Geometry check sheet. Reference: the model listing, model coordinates, mm. Face numbers are marked on the shaded views. A direction names the side the tool comes from. Give positions to 0.01 mm unless a question says otherwise; leave off trailing zeros. Loops run counter-clockwise (first coordinate to the right, second up) from the corner with the lowest first, then second, coordinate; pieces in that order, holes last.
```python
from build123d import *

# Parameters (mm, degrees)
SKETCH1_R                      = 9.525
BOSS_EXTRUDE1_DEPTH            = 80.9625
SKETCH2_R                      = 19.05
BOSS_EXTRUDE2_DEPTH            = 4.7498
SKETCH5_OUTSIDE_W              = 60.348
SKETCH5_OUTSIDE_H              = 60.348
SKETCH5_OUTSIDE_R              = 8.4328
CUT_EXTRUDE1_DEPTH             = 12.954
SKETCH7_R                      = 12.7
BOSS_EXTRUDE3_DEPTH            = 3.175
F_8_32_TAPPED_HOLE1_AT_2_COUNT = 2
F_8_32_TAPPED_HOLE1_AT_2_PITCH = 12.7
F_8_32_TAPPED_HOLE1_AT_3_COUNT = 2
F_8_32_TAPPED_HOLE1_AT_3_PITCH = 21.997045256
F_8_32_TAPPED_HOLE1_AT_4_COUNT = 2
F_8_32_TAPPED_HOLE1_AT_4_PITCH = 25.4
F_8_32_TAPPED_HOLE1_AT_5_COUNT = 2
F_8_32_TAPPED_HOLE1_AT_5_PITCH = 21.997045256
F_8_32_TAPPED_HOLE1_AT_6_COUNT = 2
F_8_32_TAPPED_HOLE1_AT_6_PITCH = 12.7
SKETCH6_R                      = 6.35
CUT_EXTRUDE2_DEPTH             = 90.846554588
SKETCH10_R                     = 9.525
SKETCH10_R_2                   = 6.35
BOSS_EXTRUDE4_DEPTH            = 47.625
F_5_8_11_TAPPED_HOLE1_D        = 13.49248
F_5_8_11_TAPPED_HOLE1_DEPTH    = 25.4
F_5_8_11_TAPPED_HOLE1_TIP      = 4.053549943
CUT_EXTRUDE3_DEPTH             = 1.5875
FILLET1_R                      = 0.79375
CHAMFER1_SIZE                  = 0.254


with BuildPart() as part:
    # Sketch1 → Boss-Extrude1 (new body)
    with BuildSketch(Plane.XY):
        Circle(SKETCH1_R)
    extrude(amount=BOSS_EXTRUDE1_DEPTH)

    # Sketch2 → Boss-Extrude2 (add)
    with BuildSketch(Plane.XY.offset(80.9625)):
        Circle(SKETCH2_R)
    extrude(amount=BOSS_EXTRUDE2_DEPTH)

    # Sketch5 outside → Cut-Extrude1 (cut)
    with BuildSketch(Plane(origin=(0, 0, 0), x_dir=(-1, 0, 0), z_dir=(0, 0, -1))):
        Rectangle(SKETCH5_OUTSIDE_W, SKETCH5_OUTSIDE_H)
        Circle(SKETCH5_OUTSIDE_R, mode=Mode.SUBTRACT)
    extrude(amount=-CUT_EXTRUDE1_DEPTH, mode=Mode.SUBTRACT)

    # Sketch7 → Boss-Extrude3 (add)
    with BuildSketch(Plane(origin=(0, 0, 71.4375), x_dir=(-1, 0, 0), z_dir=(0, 0, -1))):
        Circle(SKETCH7_R)
    extrude(amount=BOSS_EXTRUDE3_DEPTH)

    # Sketch8 → #8-32 Tapped Hole1 (revolve, cut)
    with BuildSketch(Plane(origin=(0, 12.7, 80.9625), x_dir=(0, 1, 0), z_dir=(1, 0, 0))):
        Polygon((0, 0), (0, 11.705806461), (1.7272, 10.668), (1.7272, 0), align=None)
    f_8_32_tapped_hole1 = revolve(axis=Axis((0, 12.7, 74.6125), (0, 0, 1)), mode=Mode.SUBTRACT)

    # #8-32 Tapped Hole1 at 2: #8-32 Tapped Hole1 ×2
    with Locations(*[Vector(-0.8660254037844382, -0.500000000000001, 0) * (i * F_8_32_TAPPED_HOLE1_AT_2_PITCH) for i in range(1, F_8_32_TAPPED_HOLE1_AT_2_COUNT)]):
        add(f_8_32_tapped_hole1, mode=Mode.SUBTRACT)

    # #8-32 Tapped Hole1 at 3: #8-32 Tapped Hole1 ×2
    with Locations(*[Vector(-0.5000000000000153, -0.8660254037844298, 0) * (i * F_8_32_TAPPED_HOLE1_AT_3_PITCH) for i in range(1, F_8_32_TAPPED_HOLE1_AT_3_COUNT)]):
        add(f_8_32_tapped_hole1, mode=Mode.SUBTRACT)

    # #8-32 Tapped Hole1 at 4: #8-32 Tapped Hole1 ×2
    with Locations(*[(0, -i * F_8_32_TAPPED_HOLE1_AT_4_PITCH, 0) for i in range(1, F_8_32_TAPPED_HOLE1_AT_4_COUNT)]):
        add(f_8_32_tapped_hole1, mode=Mode.SUBTRACT)

    # #8-32 Tapped Hole1 at 5: #8-32 Tapped Hole1 ×2
    with Locations(*[Vector(0.4999999999999846, -0.8660254037844476, 0) * (i * F_8_32_TAPPED_HOLE1_AT_5_PITCH) for i in range(1, F_8_32_TAPPED_HOLE1_AT_5_COUNT)]):
        add(f_8_32_tapped_hole1, mode=Mode.SUBTRACT)

    # #8-32 Tapped Hole1 at 6: #8-32 Tapped Hole1 ×2
    with Locations(*[Vector(0.86602540378443, -0.5000000000000151, 0) * (i * F_8_32_TAPPED_HOLE1_AT_6_PITCH) for i in range(1, F_8_32_TAPPED_HOLE1_AT_6_COUNT)]):
        add(f_8_32_tapped_hole1, mode=Mode.SUBTRACT)

    # Sketch6 → Cut-Extrude2 (cut, through all)
    with BuildSketch(Plane(origin=(0, 0, 0), x_dir=(-1, 0, 0), z_dir=(0, 0, -1))):
        Circle(SKETCH6_R)
    extrude(amount=-CUT_EXTRUDE2_DEPTH, mode=Mode.SUBTRACT)

    # Sketch10 → Boss-Extrude4 (add)
    with BuildSketch(Plane.XY.offset(85.7123)):
        with Locations(Location((0, 0, 0), (0, 0, 180))):
            Circle(SKETCH10_R)
        with Locations(Location((0, 0, 0), (0, 0, 180))):
            Circle(SKETCH10_R_2, mode=Mode.SUBTRACT)
    extrude(amount=BOSS_EXTRUDE4_DEPTH)

    # 5/8-11 Tapped Hole1
    with Locations(Plane.XY.offset(133.3373)):
        with Locations((0, 0)):
            Hole(F_5_8_11_TAPPED_HOLE1_D / 2, depth=F_5_8_11_TAPPED_HOLE1_DEPTH)
            with Locations((0, 0, -(F_5_8_11_TAPPED_HOLE1_DEPTH + F_5_8_11_TAPPED_HOLE1_TIP / 2))):  # 118° drill point
                Cone(0, F_5_8_11_TAPPED_HOLE1_D / 2, F_5_8_11_TAPPED_HOLE1_TIP, mode=Mode.SUBTRACT)

    # Sketch13 → Cut-Extrude3 (cut)
    with BuildSketch(Plane(origin=(0, 0, 0), x_dir=(-1, 0, 0), z_dir=(0, 0, -1))):
        with BuildLine():
            Line((-0.79375, -6.604), (-0.79375, 6.604))
            ThreePointArc((-0.79375, 6.604), (0, 7.39775), (0.79375, 6.604))
            Line((0.79375, 6.604), (0.79375, -6.604))
            ThreePointArc((0.79375, -6.604), (0, -7.39775), (-0.79375, -6.604))
        make_face()
    extrude(amount=-CUT_EXTRUDE3_DEPTH, mode=Mode.SUBTRACT)

    # Fillet1
    # the kernel refuses this fillet: 0.79375 mm, written as the material it takes off along each edge
    with BuildSketch(Plane(origin=(0.79375, -6.300195309, 1.5875), x_dir=(0.9853201649720871, 0.17071664388506244, 0), z_dir=(0, 0, -1)), Plane(origin=(-0.79375, 6.300195309, 1.5875), x_dir=(-0.9853201649720869, -0.17071664388506383, 0), z_dir=(0, 0, -1))) as fillet1_piece_1:
        with BuildLine():
            CenterArc((0.623581926, 0.792901977), FILLET1_R, 203.344606785, 64.006660147)
            Line((-0.105190236, 0.478370264), (-0.178067452, 0.446917093))
            ThreePointArc((-0.178067452, 0.446917093), (-0.130074305, 0.285794254), (-0.078209788, -0.013550634))
            Line((-0.078209788, -0.013550634), (0.003668129, -0.079290198))
            ThreePointArc((0.003668129, -0.079290198), (0.293450318, -0.072590818), (0.583232507, -0.079290198))
            Line((0.583232507, -0.079290198), (0.586900636, 0))
        make_face()
    extrude(amount=3.054751591, mode=Mode.SUBTRACT)
    with BuildSketch(Plane(origin=(0.79375, 6.300195309, 1.5875), x_dir=(0.985320164972087, -0.17071664388506264, 0), z_dir=(0, 0, -1)), Plane(origin=(-0.79375, -6.300195309, 1.5875), x_dir=(-0.9853201649720869, 0.17071664388506363, 0), z_dir=(0, 0, -1))) as fillet1_piece_2:
        with BuildLine():
            CenterArc((0.623581926, -0.792901977), FILLET1_R, 92.648733068, 64.006660147)
            Line((-0.105190236, -0.478370264), (-0.178067452, -0.446917093))
            ThreePointArc((-0.178067452, -0.446917093), (-0.130074305, -0.285794254), (-0.078209788, 0.013550634))
            Line((-0.078209788, 0.013550634), (0.003668129, 0.079290198))
            ThreePointArc((0.003668129, 0.079290198), (0.293450318, 0.072590818), (0.583232507, 0.079290198))
            Line((0.583232507, 0.079290198), (0.586900636, 0))
        make_face()
    extrude(amount=3.054751591, mode=Mode.SUBTRACT)

    # Chamfer1
    chamfer1_edges = [part.edges().sort_by_distance(p)[0] for p in [
        (6.35, 0, 0),
        (-4.951511004, 3.975555153, 0),
        (0, -7.39775, 0),
        (0, 7.39775, 0),
        (0.987374997, 6.408680157, 0),
        (-0.987374997, 6.408680157, 0),
        (-0.987374997, -6.408680157, 0),
        (0.987374997, -6.408680157, 0),
    ]]
    chamfer(chamfer1_edges, length=CHAMFER1_SIZE)


solid = part.part
```
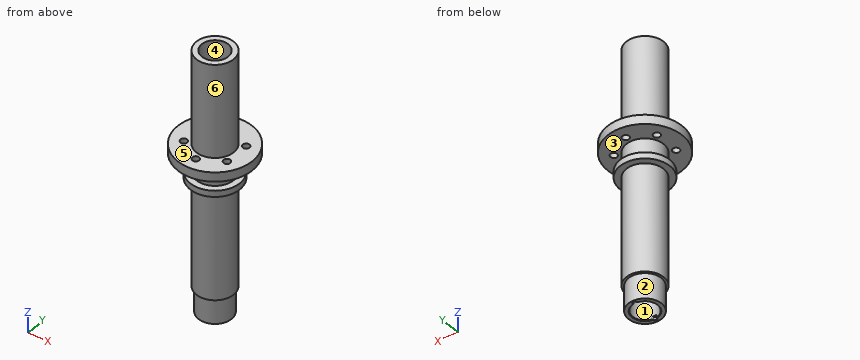
1) Mould release check, pull along X, two halves, no side actions. Record for the marked faces 4, 5 and 6: +X half, -X half, draft (parallel to the pull), parting line (faces both ways), or undercut.
2) Sectioned sample at B-B on z = 66. Enter the section's corners in (x, y) (3 decimals), plus the area to 3 significant figures.
3) Tool access check on the marked faces 1, 2 and 3. Record the directions out of +Z, -Z, +X, -X, +Y, -Y that give a thin tool (end or side, any length) a straight path to the whole face; none if there is none.
4) Scan lines: line 1 along Z through (x, y) = (-6.5, -8); line 2 along Y through (x, z) = (0, 82); line 3 along Y through (x, z) = (-1.5, 95). Record each from-to range of solid material in increasing order.
5) Depth check by flat-ended pin: P1, Ø6, axis at x = -6.5, z = 85, coming from the +Y side; P2, Ø12, axis at x = 11.5, y = -14.5, coming from the +Z side; P3, Ø3, axis at x = -11, y = -6.35, coming from the +Z side. Enter the tip coordinate at first touch or a pass-through.
6) Sectioned sample at A-A on z = 117. Enter the section's corners in (x, y) (3 decimals).
Determined:
1. face 4: undercut
1. face 5: draft
1. face 6: parting line
2. outline: circle Ø19.05 at (0, 0); hole circle Ø12.7 at (0, 0)
2. area: 158 mm2
3. face 1: +Z, -Z
3. face 2: -Z
3. face 3: none
4. line 1: z = 68.26 to 71.44, 80.96 to 85.71
4. line 2: y = -19.05 to -14.43, -10.97 to -6.35, 6.35 to 10.97, 14.43 to 19.05
4. line 3: y = -9.41 to -6.17, 6.17 to 9.41
5. P1: stops at y = 18.73
5. P2: stops at z = 85.71
5. P3: stops at z = 71.44
6. outline: circle Ø19.05 at (0, 0); hole circle Ø13.492 at (0, 0)
